```python
from build123d import *

# Parameters (mm, degrees)
SKETCH5_W           = 30
SKETCH5_H           = 30
BOSS_EXTRUDE1_DEPTH = 5
SKETCH5_3_W         = 5
SKETCH5_3_H         = 5
BOSS_EXTRUDE2_DEPTH = 150
CUT_EXTRUDE2_REACH  = 148.544
SKETCH6_R           = 2.5


with BuildPart() as part:
    # Sketch5 → Boss-Extrude1 (new body)
    with BuildSketch(Plane(origin=(0, 0, 0), x_dir=(1, 0, 0), z_dir=(0, 1, 0))):
        Rectangle(SKETCH5_W, SKETCH5_H)
    extrude(amount=BOSS_EXTRUDE1_DEPTH)

    # Sketch5_3 → Boss-Extrude2 (add)
    with BuildSketch(Plane(origin=(0, 0, 0), x_dir=(1, 0, 0), z_dir=(0, 1, 0))):
        Rectangle(SKETCH5_3_W, SKETCH5_3_H)
    extrude(amount=BOSS_EXTRUDE2_DEPTH)

    # Sketch6 → Cut-Extrude2 (cut, up to next)
    with BuildSketch(Plane(origin=(0, 5, 0), x_dir=(1, 0, 0), z_dir=(0, 1, 0)), mode=Mode.PRIVATE) as cut_extrude2_sk1:
        with Locations(Location((0, 10, 0), (0, 0, 270))):
            Circle(SKETCH6_R)
    cut_extrude2_tool1 = extrude(cut_extrude2_sk1.sketch, amount=-CUT_EXTRUDE2_REACH, mode=Mode.PRIVATE) & part.part
    # Sketch6 → Cut-Extrude2 (cut, up to next)
    with BuildSketch(Plane(origin=(0, 5, 0), x_dir=(1, 0, 0), z_dir=(0, 1, 0)), mode=Mode.PRIVATE) as cut_extrude2_sk2:
        with Locations(Location((10, 0, 0), (0, 0, 270))):
            Circle(SKETCH6_R)
    cut_extrude2_tool2 = extrude(cut_extrude2_sk2.sketch, amount=-CUT_EXTRUDE2_REACH, mode=Mode.PRIVATE) & part.part
    # Sketch6 → Cut-Extrude2 (cut, up to next)
    with BuildSketch(Plane(origin=(0, 5, 0), x_dir=(1, 0, 0), z_dir=(0, 1, 0)), mode=Mode.PRIVATE) as cut_extrude2_sk3:
        with Locations(Location((0, -10, 0), (0, 0, 270))):
            Circle(SKETCH6_R)
    cut_extrude2_tool3 = extrude(cut_extrude2_sk3.sketch, amount=-CUT_EXTRUDE2_REACH, mode=Mode.PRIVATE) & part.part
    # Sketch6 → Cut-Extrude2 (cut, up to next)
    with BuildSketch(Plane(origin=(0, 5, 0), x_dir=(1, 0, 0), z_dir=(0, 1, 0)), mode=Mode.PRIVATE) as cut_extrude2_sk4:
        with Locations(Location((-10, 0, 0), (0, 0, 270))):
            Circle(SKETCH6_R)
    cut_extrude2_tool4 = extrude(cut_extrude2_sk4.sketch, amount=-CUT_EXTRUDE2_REACH, mode=Mode.PRIVATE) & part.part
    add(cut_extrude2_tool1.solids().sort_by_distance((0, 5, -10))[0], mode=Mode.SUBTRACT)
    add(cut_extrude2_tool2.solids().sort_by_distance((10, 5, 0))[0], mode=Mode.SUBTRACT)
    add(cut_extrude2_tool3.solids().sort_by_distance((0, 5, 10))[0], mode=Mode.SUBTRACT)
    add(cut_extrude2_tool4.solids().sort_by_distance((-10, 5, 0))[0], mode=Mode.SUBTRACT)


solid = part.part
```
For this review, take the finished solid that the model builds, in its own axes (mm). A direction names the side the tool comes from. Give positions to 0.01 mm unless a question says otherwise; leave off trailing zeros. Write each loop counter-clockwise with the first axis right and the second up, starting at its lowest first coordinate (ties: lowest second). Pieces come first, ordered by that corner, then holes. Notation, with made-up numbers: M 1.25,12 L 44.25,12 A26 ccw 44.25,31 Z; hole C 75,-28 d1. An arc over 180 degrees is marked long. Answer as CSV lines item,"result".
1. Consider section A-A, the plane x = 10. Write out the cut boundary in (y, z), then the cut area to 3 significant figures.
Findings:
outline,"M 0,-15 L 5,-15 L 5,-2.5 L 0,-2.5 Z; M 0,2.5 L 5,2.5 L 5,15 L 0,15 Z"
area,"125 mm2"
2. Consider section D-D, the plane y = 40.5. Write out the cut boundary in (x, z), then the cut area to 3 significant figures.
Findings:
outline,"M -2.5,-2.5 L 2.5,-2.5 L 2.5,2.5 L -2.5,2.5 Z"
area,"25.0 mm2"
3. Wall thickness on line 1 (X direction, y = 4.05, z = 0); line 2 (X direction, y = 3.4, z = 10); line 3 (X direction, y = 119.5, z = -1): over which ranges is each line inside the solid? List them lowest first.
Findings:
line 1,"x = -15 to -12.5, -7.5 to 7.5, 12.5 to 15"
line 2,"x = -15 to -2.5, 2.5 to 15"
line 3,"x = -2.5 to 2.5"
4. For faces 1 (the flat face through (0, 76, 2.5)), 2 (the flat face through (0, 76, -2.5)), 3 (the flat face through (2.5, 76, 0)), list the 3-axis set-ups (+Z, -Z, +X, -X, +Y, -Y) from which the entire face can be reached by the end or side of a thin tool; tool diameter is ignored.
Findings:
face 1,"+Z, +X, -X, +Y"
face 2,"-Z, +X, -X, +Y"
face 3,"+Z, -Z, +X, +Y"
5. Draft analysis for pull direction X (two halves, no side actions). For faces 4 (the flat face through (-4, 5, 0)), 5 (the flat face through (-15, 2, 0)), 6 (the cylindrical face through (-12.44, 2.54, -0.54)), 7 (the cylindrical face through (0.1, 2.5, 7.5)), state which applies: +X half, -X half, draft (parallel to the pull), parting line (faces both ways), or undercut.
Findings:
face 4,"draft"
face 5,"-X half"
face 6,"undercut"
face 7,"undercut"
6. Consider section B-B, the plane z = 10. Write out the cut boundary in (x, y), then the cut area to 3 significant figures.
Findings:
outline,"M -15,0 L -2.5,0 L -2.5,5 L -15,5 Z; M 2.5,0 L 15,0 L 15,5 L 2.5,5 Z"
area,"125 mm2"
7. For pin 1 (10 mm diameter, centred on x = 3.5, y = 65.5, fed in from +Z); pin 2 (4 mm diameter, centred on x = -10, z = 0, fed in from +Y); pin 3 (1 mm diameter, centred on x = 11.5, z = 11, fed in from -Y); pin 4 (1 mm diameter, centred on x = 2, y = 108.5, fed in from -Z), all flat-tipped, find the tip position at first contact; note any pin that passes through.
Findings:
pin 1,"stops at z = 2.5"
pin 2,"passes through"
pin 3,"stops at y = 0"
pin 4,"stops at z = -2.5"
8. Consider section C-C, the plane z = -1. Write out the cut boundary in (x, y), then the cut area to 3 significant figures.
Findings:
outline,"M -15,0 L -12.29,0 L -12.29,5 L -15,5 Z; M -7.71,0 L 7.71,0 L 7.71,5 L 2.5,5 L 2.5,150 L -2.5,150 L -2.5,5 L -7.71,5 Z; M 12.29,0 L 15,0 L 15,5 L 12.29,5 Z"
area,"829 mm2"
